Check sheet for the modelled part. Datum: model origin and axes. Units: mm. Face numbers are marked on the shaded views. A direction names the side the tool comes from. Round coordinates to 2 decimals unless told otherwise and drop trailing zeros. Loops run counter-clockwise (first coordinate to the right, second up) from the corner with the lowest first, then second, coordinate; pieces in that order, holes last. Notation, with made-up numbers: (34, -12.5) -> (93, -12.5) arc R35 ccw to (93, 26.5) -> close; hole circle Ø3 at (-31.75, -3.5). An arc over 180 degrees is marked (long way). Return JSON: item names as keys, results as strings.
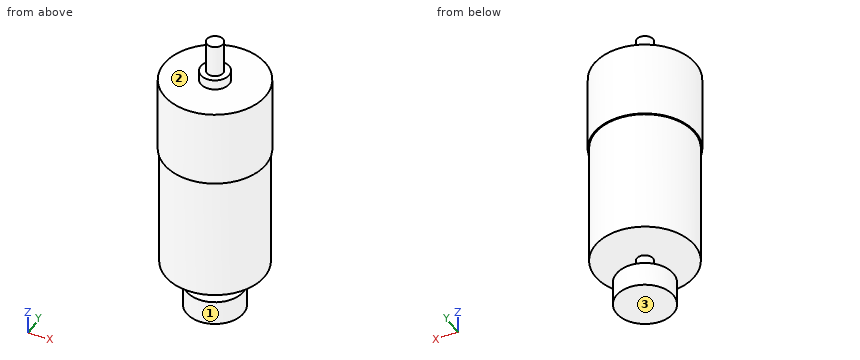
from build123d import *

# Parameters (mm, degrees)
CROQUIS1_R              = 12.5
SALIENTE_EXTRUIR1_DEPTH = 19
CROQUIS3_R              = 3.5
SALIENTE_EXTRUIR2_DEPTH = 2.5
CROQUIS4_R              = 2
SALIENTE_EXTRUIR3_DEPTH = 8
CROQUIS5_R              = 12.2
SALIENTE_EXTRUIR4_DEPTH = 31
SALIENTE_EXTRUIR5_START = 6
CROQUIS6_R              = 2
SALIENTE_EXTRUIR5_DEPTH = 6
CROQUIS7_R              = 7
SALIENTE_EXTRUIR6_DEPTH = 6


with BuildPart() as part:
    # Croquis1 → Saliente-Extruir1 (new body)
    with BuildSketch(Plane.XY):
        Circle(CROQUIS1_R)
    extrude(amount=SALIENTE_EXTRUIR1_DEPTH)

    # Croquis3 → Saliente-Extruir2 (add)
    with BuildSketch(Plane.XY.offset(19)):
        Circle(CROQUIS3_R)
    extrude(amount=SALIENTE_EXTRUIR2_DEPTH)

    # Croquis4 → Saliente-Extruir3 (add)
    with BuildSketch(Plane.XY.offset(21.5)):
        Circle(CROQUIS4_R)
    extrude(amount=SALIENTE_EXTRUIR3_DEPTH)

    # Croquis5 → Saliente-Extruir4 (add)
    with BuildSketch(Plane(origin=(0, 0, 0), x_dir=(-1, 0, 0), z_dir=(0, 0, -1))):
        Circle(CROQUIS5_R)
    extrude(amount=SALIENTE_EXTRUIR4_DEPTH)

    # Croquis6 → Saliente-Extruir5 (add)
    with BuildSketch(Plane(origin=(0, 0, -31), x_dir=(-1, 0, 0), z_dir=(0, 0, -1)).offset(SALIENTE_EXTRUIR5_START)):
        with Locations(Location((0, 0, 0), (0, 0, 180))):
            Circle(CROQUIS6_R)
    extrude(amount=-SALIENTE_EXTRUIR5_DEPTH)

    # Croquis7 → Saliente-Extruir6 (add)
    with BuildSketch(Plane(origin=(0, 0, -37), x_dir=(-1, 0, 0), z_dir=(0, 0, -1))):
        Circle(CROQUIS7_R)
    extrude(amount=SALIENTE_EXTRUIR6_DEPTH)


solid = part.part
Q1. Section check B-B (x = 6). Record the boundary of the cut face in (y, z).
Results list:
{"outline": "(-10.97, 0) -> (-10.62, 0) -> (-10.62, -31) -> (10.62, -31) -> (10.62, 0) -> (10.97, 0) -> (10.97, 19) -> (-10.97, 19) -> close; (-3.61, -43) -> (3.61, -43) -> (3.61, -37) -> (-3.61, -37) -> close"}
Q2. Tool access check on the marked faces 1, 2 and 3. Record the directions out of +Z, -Z, +X, -X, +Y, -Y that give a thin tool (end or side, any length) a straight path to the whole face; none if there is none.
Results list:
{"face 1": "-Z", "face 2": "+Z", "face 3": "-Z, +X, -X, +Y, -Y"}
Q3. Section check A-A (y = -6.25). Record the boundary of the cut face in (x, z), then the cut area to 3 significant figures.
Results list:
{"outline": "(-10.83, 0) -> (-10.48, 0) -> (-10.48, -31) -> (10.48, -31) -> (10.48, 0) -> (10.83, 0) -> (10.83, 19) -> (-10.83, 19) -> close; (-3.15, -43) -> (3.15, -43) -> (3.15, -37) -> (-3.15, -37) -> close", "area": "1,100 mm^2"}
Q4. Go/stop test with flat-tipped pins: pin 1 (6 mm diameter, centred on y = 1.5, z = -20, fed in from -X); pin 2 (12 mm diameter, centred on x = -4, z = 11.5, fed in from +Y); pin 3 (1 mm diameter, centred on x = -8.5, y = 1.5, fed in from -Z); pin 4 (1 mm diameter, centred on y = 3, z = -4.5, fed in from +X). Record where each tip stops, or that it passes through.
Results list:
{"pin 1": "x = -12.2", "pin 2": "y = 12.5", "pin 3": "z = -31", "pin 4": "x = 11.94"}
Q5. Section check C-C (y = 0). Record the boundary of the cut face in (x, z), then the cut area to 3 significant figures.
Results list:
{"outline": "(-12.5, 0) -> (-12.2, 0) -> (-12.2, -31) -> (-2, -31) -> (-2, -37) -> (-7, -37) -> (-7, -43) -> (7, -43) -> (7, -37) -> (2, -37) -> (2, -31) -> (12.2, -31) -> (12.2, 0) -> (12.5, 0) -> (12.5, 19) -> (3.5, 19) -> (3.5, 21.5) -> (2, 21.5) -> (2, 29.5) -> (-2, 29.5) -> (-2, 21.5) -> (-3.5, 21.5) -> (-3.5, 19) -> (-12.5, 19) -> close", "area": "1,390 mm^2"}
Q6. Material ranges on line 1 (Z direction, x = 4.5, y = -2.5); line 2 (Z direction, x = -9.5, y = -5.5); line 3 (Y direction, x = 10, z = -12), recorded low to high.
Results list:
{"line 1": "-43 to -37, -31 to 19", "line 2": "-31 to 19", "line 3": "-6.99 to 6.99"}
